The figure shows three views and two pictorial views of one solid part (mm, origin at its lowest corner). Answer the questions. Round coordinates to 2 decimals unless told otherwise and drop trailing zeros. Write each loop counter-clockwise with the first axis right and the second up, starting at its lowest first coordinate (ties: lowest second). Pieces come first, ordered by that corner, then holes. Notation, with made-up numbers: (-16, 14) - (-12, 14) arc R9 cw to (-12, 20) - close; hole circle Ø4 at (65.25, -27.5). An arc over 180 degrees is marked (long way). Answer as CSV lines item,"result". Start each with the question number.
Item 1: For a pull along X with two mould halves and no side action, classify the marked faces 1, 2 and 3 as pulls with the +X half, pulls with the -X half, needs draft (parallel to the pull), parting line crosses it, or undercut.
Item 2: Straight lines are drawn through the part: line 1 along Y through (x, z) = (6.75, 2.5); line 2 along Y through (x, z) = (17, 3.05); line 3 along Y through (x, z) = (3.5, 2.85). For each, find the intervals that lie inside material, in ascending order. Write a range as [from, to].
Item 3: A cutting plane is placed at C-C on z = 2.5. Determine the outline of the cut face in (x, y), and give its area (3 significant figures).
Item 4: A cutting plane is placed at D-D on y = 6. Determine the outline of the cut face in (x, z), and give its area (3 significant figures).
Item 5: A cutting plane is placed at A-A on x = 17. Determine the outline of the cut face in (y, z), and give its area (4 significant figures).
Item 6: Flat-ended cylindrical pins translate along their axes: pin 1 (0.6 mm diameter, centred on y = 5.5, z = 2.5, fed in from -X); pin 2 (1.5 mm diameter, centred on x = 11, z = 3, fed in from -Y); pin 3 (1.2 mm diameter, centred on y = 6, z = 2.5, fed in from +X). Find the tip coordinate at first contact, or state that the pin passes through.
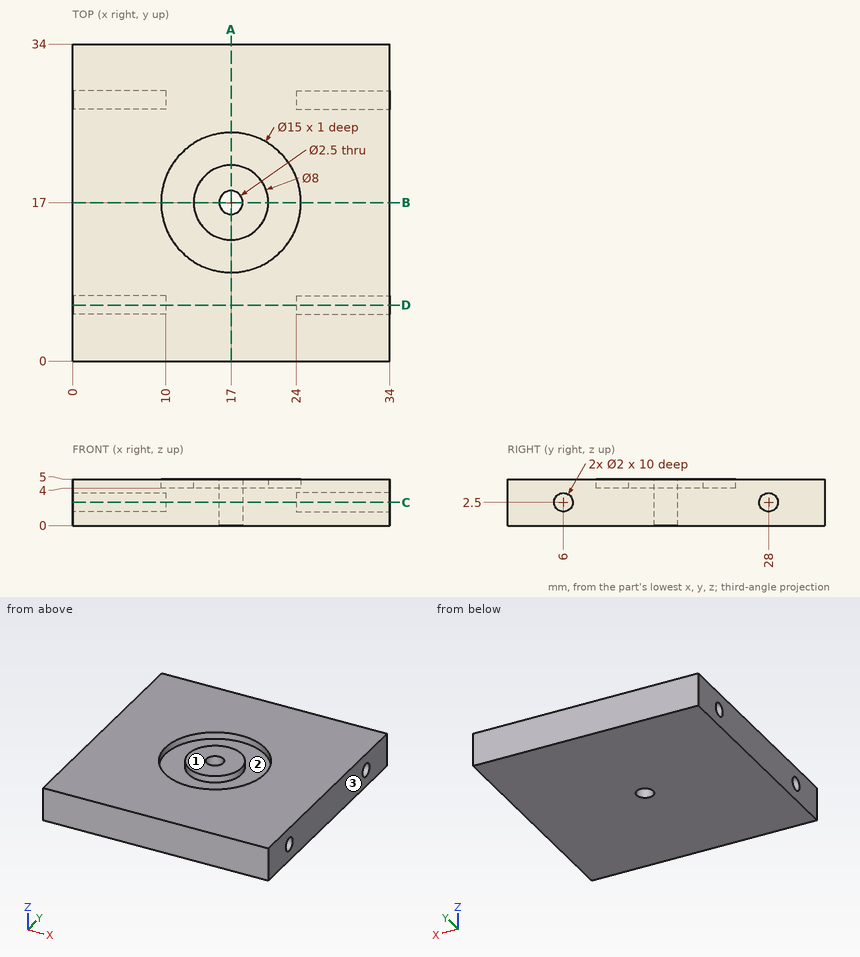
Geometry says:
1,face 1,"needs draft"
1,face 2,"undercut"
1,face 3,"pulls with the +X half"
2,line 1,"y = [0, 5], [7, 27], [29, 34]"
2,line 2,"y = [0, 15.75], [18.25, 34]"
2,line 3,"y = [0, 5.06], [6.94, 27.06], [28.94, 34]"
3,outline,"(0, 0) - (34, 0) - (34, 5) - (24, 5) - (24, 7) - (34, 7) - (34, 27) - (24, 27) - (24, 29) - (34, 29) - (34, 34) - (0, 34) - (0, 29) - (10, 29) - (10, 27) - (0, 27) - (0, 7) - (10, 7) - (10, 5) - (0, 5) - close; hole circle Ø2.5 at (17, 17)"
3,area,"1,070 mm^2"
4,outline,"(0, 0) - (34, 0) - (34, 1.5) - (24, 1.5) - (24, 3.5) - (34, 3.5) - (34, 5) - (0, 5) - (0, 3.5) - (10, 3.5) - (10, 1.5) - (0, 1.5) - close"
4,area,"130 mm^2"
5,outline,"(0, 0) - (15.75, 0) - (15.75, 5) - (13, 5) - (13, 4) - (9.5, 4) - (9.5, 5) - (0, 5) - close; (18.25, 0) - (34, 0) - (34, 5) - (24.5, 5) - (24.5, 4) - (21, 4) - (21, 5) - (18.25, 5) - close"
5,area,"150.5 mm^2"
6,pin 1,"stops at x = 10"
6,pin 2,"stops at y = 0"
6,pin 3,"stops at x = 24"
